```python
from build123d import *

# Parameters (mm, degrees)
F0_W     = 155.9993997216
F0_H     = 92.4738738686
F1_DEPTH = 80.01
F2_W     = 95.3351967037
F2_H     = 32.017163316
F3_DEPTH = 111.5057298372
F4_R     = 12.3144153275
F5_DEPTH = 174.76321174


with BuildPart() as f1:
    # F0 (on Top) → F1 (new body)
    with BuildSketch(Plane.XY):
        Polygon((-75.7883712649, 77.9326930642), (-85.4378119111, 77.9326930642), (-85.4378119111, 68.2832449675), (-85.4378119111, -24.1906289011), (-85.4378119111, -33.572036773), (80.2110284567, -33.572036773), (89.3243998289, -33.572036773), (89.3243998289, -24.1906289011), (89.3243998289, 68.2832449675), (89.3243998289, 77.9326930642), align=None)
        with Locations((2.2113285959, 22.0463080332)):
            Rectangle(F0_W, F0_H, mode=Mode.SUBTRACT)
    extrude(amount=F1_DEPTH)

    # F2 (on face) → F3 (cut, through all)
    with BuildSketch(Plane.XZ.offset(33.572036773)):
        with Locations((2.1493490785, 64.001418342)):
            Rectangle(F2_W, F2_H)
    extrude(amount=-F3_DEPTH, mode=Mode.SUBTRACT)

    # F4 (on face) → F5 (cut, through all)
    with BuildSketch(Plane.YZ.offset(89.3243998289)):
        with Locations((20.1669149101, 42.7727550268)):
            Circle(F4_R)
    extrude(amount=-F5_DEPTH, mode=Mode.SUBTRACT)


solid = f1.part
```
For this review, take the finished solid that the model builds, in its own axes (mm). A direction names the side the tool comes from. Round coordinates to 2 decimals unless told otherwise and drop trailing zeros. Order: outer loops, then holes, each group sorted by start corner. A loop starts at its lowest first (then second) coordinate and runs counter-clockwise, first axis right, second up.
Q1. We need section A-A, the plane x = 52.5. Give the boundary of the cut face in (y, z), plus the area to 3 significant figures.
Findings below:
outline: (-33.57, 0) - (-24.19, 0) - (-24.19, 80.01) - (-33.57, 80.01) - close; (68.28, 0) - (77.93, 0) - (77.93, 80.01) - (68.28, 80.01) - close
area: 1,520 mm2
Q2. Mouldability with a two-part tool opening along Z and no side actions: class faces 4 (the cylindrical face through (-80.55, 17.5, 30.75)), 5 (the flat face through (80.211, 32, 31)), 6 (the flat face through (1, -29, 47.993)) as pulls with the +Z half, pulls with the -Z half, needs draft (parallel to the pull), parting line crosses it, or undercut.
Findings below:
face 4: undercut
face 5: needs draft
face 6: pulls with the +Z half
Q3. Wall thickness on line 1 (Y direction, x = -63.5, z = 21.5); line 2 (X direction, y = 65, z = 11); line 3 (X direction, y = -26, z = 58.5): over which ranges is each line inside the solid? List them lowest first.
Findings below:
line 1: y = -33.57 to -24.19, 68.28 to 77.93
line 2: x = -85.44 to -75.79, 80.21 to 89.32
line 3: x = -85.44 to -45.52, 49.82 to 89.32
Q4. Insertion check: P1, Ø3, axis at x = -5.5, y = 72, coming from the +Z side. The pin has a flat end and moves straight along its axis. Give the tip position at first contact, or say it passes through.
Findings below:
P1: stops at z = 47.99
Q5. We need section B-B, the plane z = 71. Give the boundary of the cut face in (x, y), plus the area to 3 significant figures.
Findings below:
outline: (-85.44, -33.57) - (-45.52, -33.57) - (-45.52, -24.19) - (-75.79, -24.19) - (-75.79, 68.28) - (-45.52, 68.28) - (-45.52, 77.93) - (-85.44, 77.93) - close; (49.82, -33.57) - (89.32, -33.57) - (89.32, 77.93) - (49.82, 77.93) - (49.82, 68.28) - (80.21, 68.28) - (80.21, -24.19) - (49.82, -24.19) - close
area: 3,250 mm2
Q6. We need section C-C, the plane y = 55. Give the boundary of the cut face in (x, z), plus the area to 3 significant figures.
Findings below:
outline: (-85.44, 0) - (-75.79, 0) - (-75.79, 80.01) - (-85.44, 80.01) - close; (80.21, 0) - (89.32, 0) - (89.32, 80.01) - (80.21, 80.01) - close
area: 1,500 mm2
Q7. Machinability: for faces 1 (the flat face through (1, 68.283, 31)), 2 (the cylindrical face through (84.83, 17.5, 30.75)), 3 (the flat face through (49.817, -29, 64)), which of the approach directions +Z, -Z, +X, -X, +Y, -Y give a long, thin tool a straight path to every point of the face, cutting with its end or side? Answer none if there is none.
Findings below:
face 1: +Z, -Z
face 2: +X, -X
face 3: +Z, +Y, -Y
Q8. We need section D-D, the plane z = 6. Give the boundary of the cut face in (x, y).
Findings below:
outline: (-85.44, -33.57) - (89.32, -33.57) - (89.32, 77.93) - (-85.44, 77.93) - close; hole (-75.79, -24.19) - (80.21, -24.19) - (80.21, 68.28) - (-75.79, 68.28) - close
